Model file for the job. Use its own axes, mm. A direction names the side the tool comes from. Coordinates: 2 decimals unless noted, no trailing zeros. Order: outer loops, then holes, each group sorted by start corner. A loop starts at its lowest first (then second) coordinate and runs counter-clockwise, first axis right, second up.
from build123d import *

# Parameters (mm, degrees)
F1_DEPTH = 2.54
F2_W     = 89.8525
F2_H     = 1.7887626846
F3_DEPTH = 50.8
F4_R     = 8.509
F4_R_2   = 0.889
F4_W     = 48.4873057247
F4_H     = 25.5061189608
F5_DEPTH = 25.4


# Not quite as in the source:
# - a feature names something its author has since deleted; it is built from what else it names


with BuildPart() as f1:
    # F0 (on Top) → F1 (new body)
    with BuildSketch(Plane.XY):
        with BuildLine():
            Line((46.9198958446, -15.3550693233), (-42.9326041554, -15.3550693233))
            Line((-42.9326041554, -15.3550693233), (-42.9326041554, -18.9255226487))
            Line((-42.9326041554, -18.9255226487), (-39.7576041554, -18.9255226487))
            ThreePointArc((-39.7576041554, -18.9255226487), (-38.4876041554, -17.6555226487), (-37.2176041554, -18.9255226487))
            Line((-37.2176041554, -18.9255226487), (41.2048958446, -18.9255226487))
            ThreePointArc((41.2048958446, -18.9255226487), (42.4748958446, -17.6555226487), (43.7448958446, -18.9255226487))
            Line((43.7448958446, -18.9255226487), (46.9198958446, -18.9255226487))
            Line((46.9198958446, -18.9255226487), (46.9198958446, -15.3550693233))
        make_face()
        with BuildLine():
            Line((-39.7576041554, -18.9255226487), (-42.9326041554, -18.9255226487))
            Line((-42.9326041554, -18.9255226487), (-42.9326041554, -28.0550693233))
            Line((-42.9326041554, -28.0550693233), (46.9198958446, -28.0550693233))
            Line((46.9198958446, -28.0550693233), (46.9198958446, -18.9255226487))
            Line((46.9198958446, -18.9255226487), (43.7448958446, -18.9255226487))
            ThreePointArc((43.7448958446, -18.9255226487), (42.4748958446, -20.1955226487), (41.2048958446, -18.9255226487))
            Line((41.2048958446, -18.9255226487), (-37.2176041554, -18.9255226487))
            ThreePointArc((-37.2176041554, -18.9255226487), (-38.4876041554, -20.1955226487), (-39.7576041554, -18.9255226487))
        make_face()
    extrude(amount=F1_DEPTH)

    # F2 (on face) → F3 (join)
    with BuildSketch(Plane.XY.offset(2.54)):
        with Locations((1.9936458446, -27.160687981)):
            Rectangle(F2_W, F2_H)
    extrude(amount=F3_DEPTH)

    # F4 (on face) → F5 (cut)
    with BuildSketch(Plane.XZ.offset(28.0550693233)):
        with Locations((-10.8520889408, 13.5200908117)):
            Circle(F4_R)
        with Locations((14.9718186097, 13.4496116212)):
            Circle(F4_R)
        with Locations((-18.9169041554, 21.9057271107)):
            Circle(F4_R_2)
        with Locations((-18.9169041554, 5.1380908117)):
            Circle(F4_R_2)
        with Locations((22.9168958446, 5.1380908117)):
            Circle(F4_R_2)
        with Locations((22.9168958446, 21.7611324307)):
            Circle(F4_R_2)
        Polygon((46.9198958446, 53.34), (26.2442958446, 53.34), (26.2442958446, 27.8338810392), (26.2442958446, 2.3277620785), (46.9198958446, 2.3277620785), align=None)
        Polygon((-22.2430098802, 53.34), (-42.9326041554, 53.34), (-42.9326041554, 2.3277620785), (-22.2430098802, 2.3277620785), (-22.2430098802, 27.8338810392), align=None)
        with Locations((2.0006429822, 40.5869405196)):
            Rectangle(F4_W, F4_H)
    extrude(amount=-F5_DEPTH, mode=Mode.SUBTRACT)


solid = f1.part
Q1. Cut at C-C, the plane z = 16.75. List the corners of the cut face in (x, y).
Established:
outline: (-22.24, -28.06) - (-18.72, -28.06) - (-18.72, -26.27) - (-22.24, -26.27) - close; (-2.98, -28.06) - (7.13, -28.06) - (7.13, -26.27) - (-2.98, -26.27) - close; (22.81, -28.06) - (26.24, -28.06) - (26.24, -26.27) - (22.81, -26.27) - close
Q2. Cut at B-B, the plane y = -25.5. List the corners of the cut face in (x, z).
Established:
outline: (-42.93, 0) - (46.92, 0) - (46.92, 2.33) - (26.24, 2.33) - (26.24, 2.54) - (-22.24, 2.54) - (-22.24, 2.33) - (-42.93, 2.33) - close
Q3. Drop flat-ended pins along their axis: P1, Ø6.5, axis at x = 34.5, y = -19, coming from the +Z side; P2, Ø3.5, axis at x = -8.5, y = -20.5, coming from the +Z side; P3, Ø3, axis at y = -26.5, z = 11, coming from the +X side. Give the stop position or say it passes through.
Established:
P1: stops at z = 2.33
P2: stops at z = 2.54
P3: stops at x = 26.24
Q4. Cut at D-D, the plane x = 11. List the corners of the cut face in (y, z).
Established:
outline: (-28.06, 0) - (-15.36, 0) - (-15.36, 2.54) - (-26.27, 2.54) - (-26.27, 5.92) - (-28.06, 5.92) - close; (-28.06, 20.97) - (-26.27, 20.97) - (-26.27, 27.83) - (-28.06, 27.83) - close
Q5. Probe line 1 (Z direction, x = 9, y = -21.25); line 2 (Z direction, x = 28.5, y = -16); line 3 (Y direction, x = -1, z = 20.25). List the from-to ranges inside material, lowest first.
Established:
line 1: z = 0 to 2.54
line 2: z = 0 to 2.33
line 3: y = -28.06 to -26.27
Q6. Which spindle directions (+Z, -Z, +X, -X, +Y, -Y) get a long thin tool onto all of the face, cutting with end or side? Do faces 5 (the face through (2, -26.266, 15)), 6 (the face through (-18.096, -27.173, 4.798)), 7 (the face through (-33, -22, 2.328)), 8 (the face through (26.244, -27, 15)). Say none if no direction does.
Established:
face 5: +Z, +X, -X, +Y
face 6: +Y, -Y
face 7: +Z, -X, +Y, -Y
face 8: +Z, +X, +Y, -Y
Q7. Cut at A-A, the plane x = -13. List the corners of the cut face in (y, z), plus the area to 3 significant figures.
Established:
outline: (-28.06, 0) - (-15.36, 0) - (-15.36, 2.54) - (-26.27, 2.54) - (-26.27, 5.29) - (-28.06, 5.29) - close; (-28.06, 21.75) - (-26.27, 21.75) - (-26.27, 27.83) - (-28.06, 27.83) - close
area: 48.0 mm2
Q8. Mould opens along Z. For faces 1 (the face through (1, -22, 0)), 2 (the face through (18.9, -27.2, 5.9)), 3 (the face through (36, -22, 2.328)), 4 (the face through (3, -15.355, 1)) say: pulls with the +Z half, pulls with the -Z half, needs draft (parallel to the pull), parting line crosses it, or undercut.
Established:
face 1: pulls with the -Z half
face 2: undercut
face 3: pulls with the +Z half
face 4: needs draft
